The drawing under review shows one solid part. Ordinate dimensions are in mm from its lowest x, y, z. A direction names the side the tool comes from. Round coordinates to 2 decimals unless told otherwise and drop trailing zeros. Loops run counter-clockwise (first coordinate to the right, second up) from the corner with the lowest first, then second, coordinate; pieces in that order, holes last. Notation, with made-up numbers: (-13, -1.5) - (-7, -1.5) arc R6 cw to (-7, 5.5) - close; hole circle Ø8 at (76, 73). An arc over 180 degrees is marked (long way). Answer as CSV lines item,"result".
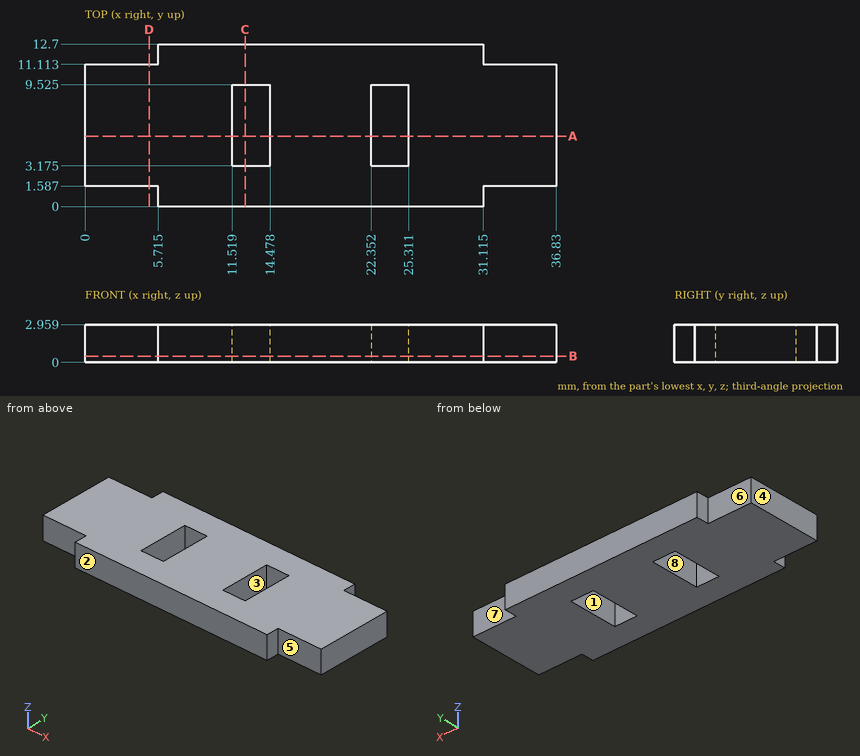
1. Take a section at B-B (z = 0.5). State the section outline as (x, y) points (1 decimal).
Numbers:
outline,"(0, 1.6) - (5.7, 1.6) - (5.7, 0) - (31.1, 0) - (31.1, 1.6) - (36.8, 1.6) - (36.8, 11.1) - (31.1, 11.1) - (31.1, 12.7) - (5.7, 12.7) - (5.7, 11.1) - (0, 11.1) - close; hole (11.5, 3.2) - (14.5, 3.2) - (14.5, 9.5) - (11.5, 9.5) - close; hole (22.4, 3.2) - (25.3, 3.2) - (25.3, 9.5) - (22.4, 9.5) - close"
2. Clearance check with flat-ended pins moving along their axes: pin 1 (0.8 mm diameter, centred on y = 0.5, z = 2, fed in from -X) (1 decimal); pin 2 (0.9 mm diameter, centred on x = 35, z = 1, fed in from +Y); pin 3 (0.5 mm diameter, centred on y = 0.5, z = 1.5, fed in from +X) (1 decimal). State where each tip first meets the part, or that it passes through.
Numbers:
pin 1,"stops at x = 5.7"
pin 2,"stops at y = 11.11"
pin 3,"stops at x = 31.1"
3. Take a section at D-D (x = 5). State the section outline as (y, z) points.
Numbers:
outline,"(1.59, 0) - (11.11, 0) - (11.11, 2.96) - (1.59, 2.96) - close"
4. Take a section at A-A (y = 5.5). State the section outline as (x, z) points.
Numbers:
outline,"(0, 0) - (11.52, 0) - (11.52, 2.96) - (0, 2.96) - close; (14.48, 0) - (22.35, 0) - (22.35, 2.96) - (14.48, 2.96) - close; (25.31, 0) - (36.83, 0) - (36.83, 2.96) - (25.31, 2.96) - close"
5. Tool access review of the marked faces 5, 6, 7 and 8: name each direction out of +Z, -Z, +X, -X, +Y, -Y from which nothing blocks a thin tool from reaching the whole face with its end or side.
Numbers:
face 5,"+Z, -Z, +X, -Y"
face 6,"+Z, -Z, -X, +Y"
face 7,"+Z, -Z, +X, +Y"
face 8,"+Z, -Z"
6. Take a section at C-C (x = 12.5). State the section outline as (y, z) points (1 decimal).
Numbers:
outline,"(0, 0) - (3.2, 0) - (3.2, 3) - (0, 3) - close; (9.5, 0) - (12.7, 0) - (12.7, 3) - (9.5, 3) - close"
7. Wall thickness on probe 1 along X at (y, z) = (6, 2.5); probe 2 along Y at (x, z) = (12, 1.1) (1 decimal); probe 3 along Y at (x, z) = (3.5, 1.1): over which ranges is each line inside the solid? List them lowest first.
Numbers:
probe 1,"x = 0 to 11.52, 14.48 to 22.35, 25.31 to 36.83"
probe 2,"y = 0 to 3.2, 9.5 to 12.7"
probe 3,"y = 1.59 to 11.11"
8. Draft analysis for pull direction X (two halves, no side actions). For the marked faces 1, 2, 3 and 4, state which applies: +X half, -X half, draft (parallel to the pull), parting line (faces both ways), or undercut.
Numbers:
face 1,"undercut"
face 2,"draft"
face 3,"undercut"
face 4,"-X half"
